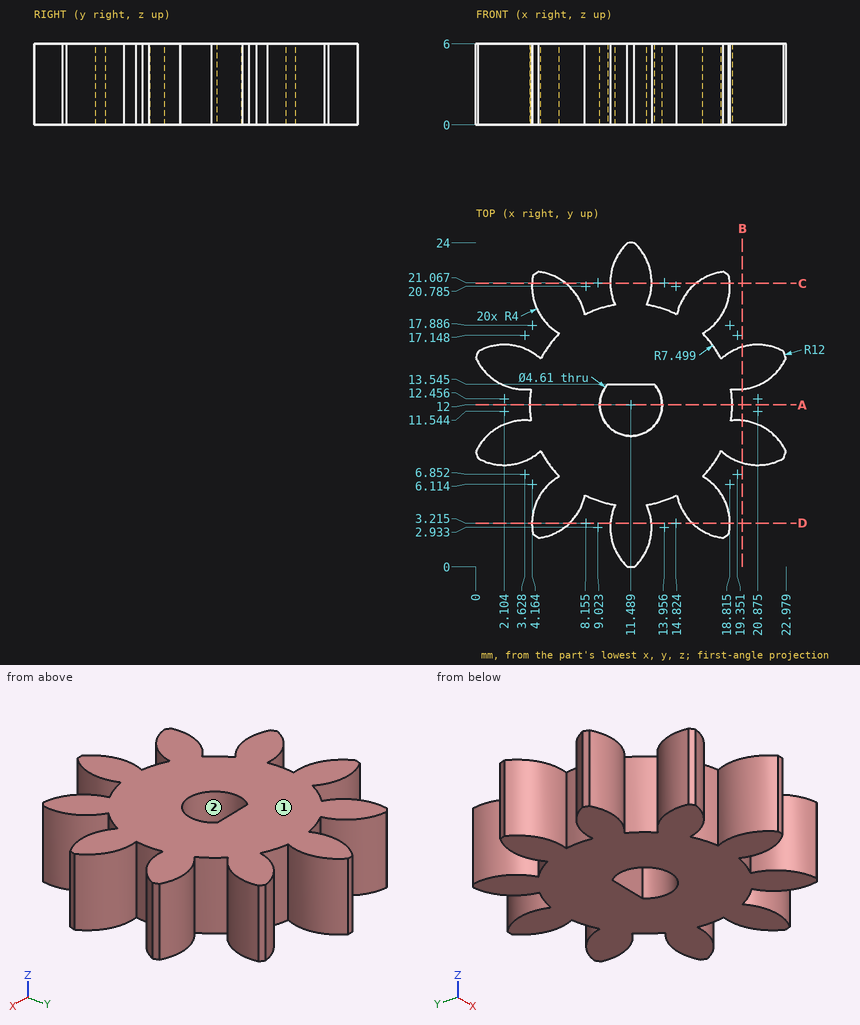
Study the drawing (mm; zero at the part's minimum x, y, z) and answer. Give positions to 0.01 mm unless a question says otherwise; leave off trailing zeros. Order: outer loops, then holes, each group sorted by start corner. A loop starts at its lowest first (then second) coordinate and runs counter-clockwise, first axis right, second up. Notation, with made-up numbers: (6.5, 87) - (23.5, 87) arc R13 cw to (23.5, 98) - close; hole circle Ø11 at (-36, 56.5). An arc over 180 degrees is marked (long way). Answer in a Markdown table with one row per item. Add a question column.
Q1. Find the intervals of material crossed by line 1 along X through (y, z) = (12, 4.25) (1 decimal); line 2 along Y through (x, z) = (1.75, 4.5) (1 decimal); line 3 along Y through (x, z) = (21.5, 1.3) (1 decimal), in increasing order. Write a range as [from, to].
Q2. The part is cut by section C-C (y = 21). Determine the outline of the cut face in (x, z) (1 decimal).
Q3. For a pull along Y with two mould halves and no side action, classify the marked faces 1 and 2 as released by +Y, released by -Y, zero draft, split by the parting line, or undercut.
Q4. The part is cut by section D-D (y = 3.25). Determine the outline of the cut face in (x, z) (1 decimal).
Q5. Given P1, Ø1.5, axis at x = 16.5, z = 4.5, coming from the +Y side; P2, Ø1, axis at y = 4, z = 3.5, coming from the +X side; P3, Ø2, axis at y = 20, z = 1.5, coming from the -X side (1 decimal), each flat-ended and moving along its own axis, determine where each tip first touches the part or whether it passes through.
Q6. The part is cut by section A-A (y = 12). Determine the outline of the cut face in (x, z) (1 decimal).
Q7. The part is cut by section B-B (x = 19.75). Determine the outline of the cut face in (y, z) (1 decimal).
Determined:
| question | item | result |
|---|---|---|
| 1 | line 1 | x = [4, 9.2], [13.8, 19] |
| 1 | line 2 | y = [7.6, 10.4], [13.6, 16.4] |
| 1 | line 3 | y = [7.6, 10.2], [13.8, 16.4] |
| 2 | outline | (4.2, 0) - (6.7, 0) - (6.7, 6) - (4.2, 6) - close; (10, 0) - (13, 0) - (13, 6) - (10, 6) - close; (16.3, 0) - (18.8, 0) - (18.8, 6) - (16.3, 6) - close |
| 3 | face 1 | zero draft |
| 3 | face 2 | undercut |
| 4 | outline | (4.2, 0) - (7, 0) - (7, 6) - (4.2, 6) - close; (10, 0) - (13, 0) - (13, 6) - (10, 6) - close; (16, 0) - (18.8, 0) - (18.8, 6) - (16, 6) - close |
| 5 | P1 | stops at y = 21.57 |
| 5 | P2 | stops at x = 18.81 |
| 5 | P3 | stops at x = 4.2 |
| 6 | outline | (4, 0) - (9.2, 0) - (9.2, 6) - (4, 6) - close; (13.8, 0) - (19, 0) - (19, 6) - (13.8, 6) - close |
| 7 | outline | (7.7, 0) - (10.8, 0) - (10.8, 6) - (7.7, 6) - close; (13.2, 0) - (16.3, 0) - (16.3, 6) - (13.2, 6) - close |
